Verification items for the finished model (mm, model axes). A direction names the side the tool comes from. Give positions to 0.01 mm unless a question says otherwise; leave off trailing zeros. Order: outer loops, then holes, each group sorted by start corner. A loop starts at its lowest first (then second) coordinate and runs counter-clockwise, first axis right, second up.
from build123d import *

# Parameters (mm, degrees)
SKETCH1_R           = 25.4
BOSS_EXTRUDE1_DEPTH = 6.35
SKETCH2_R           = 4.8641
CUT_EXTRUDE1_DEPTH  = 37.477972806
SKETCH3_R           = 5.7404
CUT_EXTRUDE3_DEPTH  = 0.8636
BOSS_EXTRUDE2_DEPTH = 6.35


with BuildPart() as part:
    # Sketch1 → Boss-Extrude1 (new body)
    with BuildSketch(Plane(origin=(0, 0, 0), x_dir=(1, 0, 0), z_dir=(0, 1, 0))):
        with Locations(Location((0, 0, 0), (0, 0, 270))):
            Circle(SKETCH1_R)
    extrude(amount=BOSS_EXTRUDE1_DEPTH)

    # Sketch2 → Cut-Extrude1 (cut, through all)
    with BuildSketch(Plane(origin=(0, 6.35, 0), x_dir=(1, 0, 0), z_dir=(0, 1, 0))):
        with Locations(Location((0, 0, 0), (0, 0, 270))):
            Circle(SKETCH2_R)
    extrude(amount=-CUT_EXTRUDE1_DEPTH, mode=Mode.SUBTRACT)

    # Sketch3 → Cut-Extrude3 (cut)
    with BuildSketch(Plane(origin=(0, 6.35, 0), x_dir=(1, 0, 0), z_dir=(0, 1, 0))):
        with Locations(Location((0, 0, 0), (0, 0, 270))):
            Circle(SKETCH3_R)
    extrude(amount=-CUT_EXTRUDE3_DEPTH, mode=Mode.SUBTRACT)

    # Sketch4 → Boss-Extrude2 (add)
    with BuildSketch(Plane(origin=(0, 6.35, 0), x_dir=(1, 0, 0), z_dir=(0, 1, 0))):
        with BuildLine():
            Line((2.921, 18.881483488), (2.921, 25.231483488))
            ThreePointArc((2.921, 25.231483488), (0, 25.4), (-2.921, 25.231483488))
            Line((-2.921, 25.231483488), (-2.921, 18.881483488))
            ThreePointArc((-2.921, 18.881483488), (0, 19.106089597), (2.921, 18.881483488))
        make_face()
        with BuildLine():
            Line((25.231483488, 2.921), (18.881483488, 2.921))
            ThreePointArc((18.881483488, 2.921), (19.106089597, 0), (18.881483488, -2.921))
            Line((18.881483488, -2.921), (25.231483488, -2.921))
            ThreePointArc((25.231483488, -2.921), (25.357835876, -1.462928468), (25.4, 0))
            ThreePointArc((25.4, 0), (25.357835876, 1.462928468), (25.231483488, 2.921))
        make_face()
    extrude(amount=BOSS_EXTRUDE2_DEPTH)


solid = part.part
(1) Release check for a two-part mould opening along X. For faces 1 (the flat face through (2.921, 9, -22)), 2 (the flat face through (-2.921, 9, -22)), 3 (the flat face through (1, 5.486, -5)) record: pulls with the +X half, pulls with the -X half, needs draft (parallel to the pull), parting line crosses it, or undercut.
Solved:
face 1: pulls with the +X half
face 2: pulls with the -X half
face 3: undercut
(2) Section check B-B, the plane z = 4. Enter the section's corners in (x, y), then the cut area to 3 significant figures.
Solved:
outline: (-25.08, 0) - (-2.77, 0) - (-2.77, 5.49) - (-4.12, 5.49) - (-4.12, 6.35) - (-25.08, 6.35) - close; (2.77, 0) - (25.08, 0) - (25.08, 6.35) - (4.12, 6.35) - (4.12, 5.49) - (2.77, 5.49) - close
area: 281 mm2
(3) Go/stop test with flat-tipped pins: pin 1 (1.5 mm diameter, centred on y = 4.5, z = 2.5, fed in from -X); pin 2 (3 mm diameter, centred on y = 8.5, z = -21, fed in from -X); pin 3 (3 mm diameter, centred on x = 18, z = 12.5, fed in from +Y). Record where each tip stops, or that it passes through.
Solved:
pin 1: stops at x = -25.34
pin 2: stops at x = -2.92
pin 3: stops at y = 6.35
(4) Set-up check for faces 4 (the cylindrical face through (-0.041, 9.481, -19.106)), 5 (the cylindrical face through (5.69, 5.92, -0.75)), 6 (the flat face through (22, 9, 2.921)): record each of +Z, -Z, +X, -X, +Y, -Y from which the full face is reachable in a straight line by a thin tool's end or side.
Solved:
face 4: +Z, +Y
face 5: +Y
face 6: +Z, +X, -X, +Y
(5) Section check A-A, the plane y = 9.25. Enter the section's corners in (x, z).
Solved:
outline: (-2.92, -25.23) arc R25.4 ccw to (2.92, -25.23) - (2.92, -18.88) arc R19.11 cw to (-2.92, -18.88) - close; (18.88, -2.92) - (25.23, -2.92) arc R25.4 ccw to (25.23, 2.92) - (18.88, 2.92) arc R19.11 cw to start
(6) Section check C-C, the plane x = 0. Enter the section's corners in (y, z), then the cut area to 3 significant figures.
Solved:
outline: (0, -25.4) - (12.7, -25.4) - (12.7, -19.11) - (6.35, -19.11) - (6.35, -5.74) - (5.49, -5.74) - (5.49, -4.86) - (0, -4.86) - close; (0, 4.86) - (5.49, 4.86) - (5.49, 5.74) - (6.35, 5.74) - (6.35, 25.4) - (0, 25.4) - close
area: 299 mm2
(7) Section check D-D, the plane y = 2.75. Enter the section's corners in (x, z), then the cut area to 3 significant figures.
Solved:
outline: circle Ø50.8 at (0, 0); hole circle Ø9.73 at (0, 0)
area: 1,950 mm2
(8) Scan lines: line 1 (X direction, y = 2.8, z = 0); line 2 (Y direction, x = -7, z = 5); line 3 (X direction, y = 5.75, z = 0). Record each from-to range of solid material in increasing order.
Solved:
line 1: x = -25.4 to -4.86, 4.86 to 25.4
line 2: y = 0 to 6.35
line 3: x = -25.4 to -5.74, 5.74 to 25.4
